from build123d import *

# Parameters (mm, degrees)
SKETCH1_W               = 19.5
SKETCH1_H               = 16
PCB_DEPTH               = 1.1
HOLES_REACH             = 14.66
SKETCH2_R               = 0.525
SKETCH3_W               = 6.970626183
SKETCH3_H               = 7.047226471
SKETCH3_W_2             = 3.232532143
SKETCH3_H_2             = 1.853726963
SKETCH3_W_3             = 1.608606043
SKETCH3_H_3             = 0.674082532
SKETCH3_H_4             = 0.766002877
SKETCH3_W_4             = 3.140611797
SKETCH3_H_5             = 1.470725524
SKETCH3_W_5             = 0.949843568
SKETCH3_H_6             = 1.363485122
SKETCH3_W_6             = 0.919203453
SKETCH3_W_7             = 1.593285985
SKETCH3_H_7             = 0.827283108
SKETCH3_W_8             = 1.577965927
SKETCH3_W_9             = 1.669886272
SKETCH3_W_10            = 1.041763914
SKETCH3_H_8             = 1.516685697
SKETCH3_W_11            = 0.93452351
BOTTOM_COMPONENTS_DEPTH = 1.05


with BuildPart() as part:
    # Sketch1 → PCB (new body)
    with BuildSketch(Plane(origin=(0, 0, 0), x_dir=(1, 0, 0), z_dir=(0, 1, 0))):
        Rectangle(SKETCH1_W, SKETCH1_H)
    extrude(amount=PCB_DEPTH)

    # Sketch2 → Holes (cut, up to next)
    with BuildSketch(Plane(origin=(0, 1.1, 0), x_dir=(1, 0, 0), z_dir=(0, 1, 0)), mode=Mode.PRIVATE) as holes_sk1:
        with Locations(Location((-8.25, -6.5, 0), (0, 0, 270))):
            Circle(SKETCH2_R)
    holes_tool1 = extrude(holes_sk1.sketch, amount=-HOLES_REACH, mode=Mode.PRIVATE) & part.part
    # Sketch2 → Holes (cut, up to next)
    with BuildSketch(Plane(origin=(0, 1.1, 0), x_dir=(1, 0, 0), z_dir=(0, 1, 0)), mode=Mode.PRIVATE) as holes_sk2:
        with Locations(Location((-8.25, -3.96, 0), (0, 0, 270))):
            Circle(SKETCH2_R)
    holes_tool2 = extrude(holes_sk2.sketch, amount=-HOLES_REACH, mode=Mode.PRIVATE) & part.part
    # Sketch2 → Holes (cut, up to next)
    with BuildSketch(Plane(origin=(0, 1.1, 0), x_dir=(1, 0, 0), z_dir=(0, 1, 0)), mode=Mode.PRIVATE) as holes_sk3:
        with Locations(Location((-8.25, -1.42, 0), (0, 0, 270))):
            Circle(SKETCH2_R)
    holes_tool3 = extrude(holes_sk3.sketch, amount=-HOLES_REACH, mode=Mode.PRIVATE) & part.part
    # Sketch2 → Holes (cut, up to next)
    with BuildSketch(Plane(origin=(0, 1.1, 0), x_dir=(1, 0, 0), z_dir=(0, 1, 0)), mode=Mode.PRIVATE) as holes_sk4:
        with Locations(Location((-8.25, 1.12, 0), (0, 0, 270))):
            Circle(SKETCH2_R)
    holes_tool4 = extrude(holes_sk4.sketch, amount=-HOLES_REACH, mode=Mode.PRIVATE) & part.part
    # Sketch2 → Holes (cut, up to next)
    with BuildSketch(Plane(origin=(0, 1.1, 0), x_dir=(1, 0, 0), z_dir=(0, 1, 0)), mode=Mode.PRIVATE) as holes_sk5:
        with Locations(Location((-8.25, 3.66, 0), (0, 0, 270))):
            Circle(SKETCH2_R)
    holes_tool5 = extrude(holes_sk5.sketch, amount=-HOLES_REACH, mode=Mode.PRIVATE) & part.part
    # Sketch2 → Holes (cut, up to next)
    with BuildSketch(Plane(origin=(0, 1.1, 0), x_dir=(1, 0, 0), z_dir=(0, 1, 0)), mode=Mode.PRIVATE) as holes_sk6:
        with Locations(Location((-8.25, 6.2, 0), (0, 0, 270))):
            Circle(SKETCH2_R)
    holes_tool6 = extrude(holes_sk6.sketch, amount=-HOLES_REACH, mode=Mode.PRIVATE) & part.part
    add(holes_tool1.solids().sort_by_distance((-8.25, 1.1, 6.5))[0], mode=Mode.SUBTRACT)
    add(holes_tool2.solids().sort_by_distance((-8.25, 1.1, 3.96))[0], mode=Mode.SUBTRACT)
    add(holes_tool3.solids().sort_by_distance((-8.25, 1.1, 1.42))[0], mode=Mode.SUBTRACT)
    add(holes_tool4.solids().sort_by_distance((-8.25, 1.1, -1.12))[0], mode=Mode.SUBTRACT)
    add(holes_tool5.solids().sort_by_distance((-8.25, 1.1, -3.66))[0], mode=Mode.SUBTRACT)
    add(holes_tool6.solids().sort_by_distance((-8.25, 1.1, -6.2))[0], mode=Mode.SUBTRACT)

    # Sketch3 → Bottom components (add)
    with BuildSketch(Plane.XZ):
        with Locations((0.666422503, 0.628122359)):
            Rectangle(SKETCH3_W, SKETCH3_H)
        with Locations((-4.43515666, -5.18583948)):
            Rectangle(SKETCH3_W_2, SKETCH3_H_2)
        with Locations((-1.034103885, -5.300739911)):
            Rectangle(SKETCH3_W_3, SKETCH3_H_3)
        with Locations((-1.034103885, -6.265903537)):
            Rectangle(SKETCH3_W_3, SKETCH3_H_4)
        with Locations((2.382268949, -6.235263421)):
            Rectangle(SKETCH3_W_4, SKETCH3_H_5)
        with Locations((4.948378587, 5.967162414)):
            Rectangle(SKETCH3_W_5, SKETCH3_H_6)
        with Locations((6.265903537, 5.967162414)):
            Rectangle(SKETCH3_W_6, SKETCH3_H_6)
        with Locations((1.945647309, 6.61826486)):
            Rectangle(SKETCH3_W_7, SKETCH3_H_7)
        with Locations((-1.325184978, 6.61826486)):
            Rectangle(SKETCH3_W_8, SKETCH3_H_7)
        with Locations((-4.481116832, 6.61826486)):
            Rectangle(SKETCH3_W_9, SKETCH3_H_7)
        with Locations((4.99433876, -5.722041494)):
            Rectangle(SKETCH3_W_10, SKETCH3_H_8)
        with Locations((6.411444083, -5.722041494)):
            Rectangle(SKETCH3_W_11, SKETCH3_H_8)
    extrude(amount=BOTTOM_COMPONENTS_DEPTH)


solid = part.part
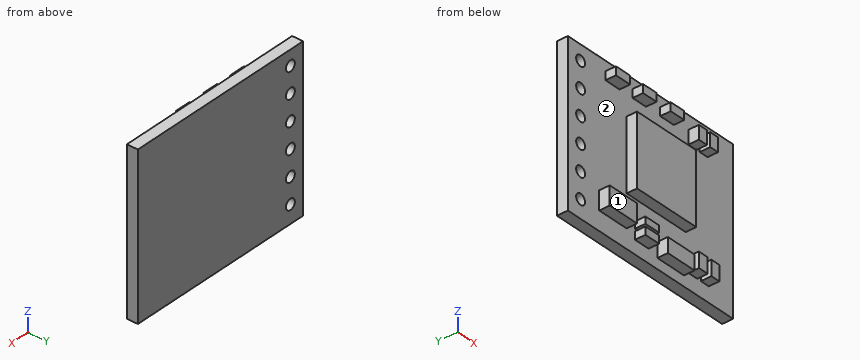
Work out the finished part from the listing and answer in its coordinate system (mm). Face numbers are marked on the shaded views. Coordinates: 2 decimals unless noted, no trailing zeros. Write each loop counter-clockwise with the first axis right and the second up, starting at its lowest first coordinate (ties: lowest second). Pieces come first, ordered by that corner, then holes. Notation, with made-up numbers: M 27,28 L 64,28 A24 ccw 64,41 Z; hole C 17,30.25 d1. An arc over 180 degrees is marked long. Answer as CSV lines item,"result". Start each with the question number.
Item 1: Section A-A on z = -1.12 is taken. Write down the section's boundary in (x, y) (3 decimals).
Item 2: Section D-D on z = -3.66 is taken. Write down the section's boundary in (x, y) (3 decimals), and give its area (3 significant figures).
Item 3: Section B-B on x = -8.25 is taken. Write down the section's boundary in (y, z) (3 decimals).
Item 4: Determine the mould class of the marked faces 1 and 2 for opening direction Z: released by +Z, released by -Z, zero draft, split by the parting line, or undercut.
Item 5: Consider L1, parallel to Z at x = 1.75, y = -0.55; L2, parallel to X at y = 0.35, z = -1.12 (3 decimals); L3, parallel to Z at x = 5.25, y = -0.7. Determine where each line is inside the solid, lowest interval first.
Item 6: Section C-C on y = 0.8 is taken. Write down the section's boundary in (x, z) (3 decimals).
Item 7: Flat-ended cylindrical pins translate along their axes: P1, Ø0.9, axis at y = -0.5, z = 6.5, coming from the +X side; P2, Ø0.5, axis at x = 5, y = -0.5, coming from the +Z side; P3, Ø0.8, axis at x = 2, y = -0.5, coming from the -Z side. Find the tip coordinate at first contact, or state that the pin passes through.
Checks:
1,outline,"M -9.75,0 L -8.775,0 L -8.775,1.1 L -9.75,1.1 Z; M -7.725,0 L -2.819,0 L -2.819,-1.05 L 4.152,-1.05 L 4.152,0 L 9.75,0 L 9.75,1.1 L -7.725,1.1 Z"
2,outline,"M -9.75,0 L -8.775,0 L -8.775,1.1 L -9.75,1.1 Z; M -7.725,0 L 9.75,0 L 9.75,1.1 L -7.725,1.1 Z"
2,area,"20.3 mm²"
3,outline,"M 0,-8 L 1.1,-8 L 1.1,-6.725 L 0,-6.725 Z; M 0,-5.675 L 1.1,-5.675 L 1.1,-4.185 L 0,-4.185 Z; M 0,-3.135 L 1.1,-3.135 L 1.1,-1.645 L 0,-1.645 Z; M 0,-0.595 L 1.1,-0.595 L 1.1,0.895 L 0,0.895 Z; M 0,1.945 L 1.1,1.945 L 1.1,3.435 L 0,3.435 Z; M 0,4.485 L 1.1,4.485 L 1.1,5.975 L 0,5.975 Z; M 0,7.025 L 1.1,7.025 L 1.1,8 L 0,8 Z"
4,face 1,"zero draft"
4,face 2,"undercut"
5,L1,"z = -6.97 to -5.5, -2.9 to 4.15, 6.2 to 7.03"
5,L2,"x = -9.75 to -8.775, -7.725 to 9.75"
5,L3,"z = -6.48 to -4.96, 5.29 to 6.65"
6,outline,"M -9.75,-8 L 9.75,-8 L 9.75,8 L -9.75,8 Z; hole C -8.25,-6.2 d1.05; hole C -8.25,-3.66 d1.05; hole C -8.25,-1.12 d1.05; hole C -8.25,1.42 d1.05; hole C -8.25,3.96 d1.05; hole C -8.25,6.5 d1.05"
7,P1,"stops at x = 6.73"
7,P2,"stops at z = 6.65"
7,P3,"stops at z = -6.97"
